Answer from the drawing. Dimensions are ordinates in mm from the lowest x, y and z of the part. Give positions to 0.01 mm unless a question says otherwise; leave off trailing zeros. Loops run counter-clockwise (first coordinate to the right, second up) from the corner with the lowest first, then second, coordinate; pieces in that order, holes last.
(1) Each of these flat-tipped pins is pushed along its axis until it touches: P1, Ø0.7, axis at x = 0.5, y = 22, coming from the +Z side (1 decimal); P2, Ø0.7, axis at x = 0.5, y = 6, coming from the +Z side (1 decimal); P3, Ø0.7, axis at x = 1, z = 22.5, coming from the -Y side. Where does it stop, or does it pass through?
(2) Find section D-D, the plane z = 25.5. Write down the section's boundary in (x, y).
(3) Find section B-B, the plane x = 0.85. State how many separate pieces and enclosed holes the cut face has, then the cut area to 3 significant figures.
(4) Find section A-A, the plane z = 15. Write down the section's boundary in (x, y), then the cut area to 3 significant figures.
(5) Straight lines are drawn through the part: probe 1 along Y at (x, z) = (0.9, 15); probe 2 along Z at (x, y) = (0.15, 6) (1 decimal); probe 3 along Y at (x, z) = (0.3, 20.5) (1 decimal). For each, find the intervals that lie inside material, in ascending order.
(6) Determine the mould class of the marked faces 1 and 2 for opening direction X: pulls with the +X half, pulls with the -X half, needs draft (parallel to the pull), parting line crosses it, or undercut.
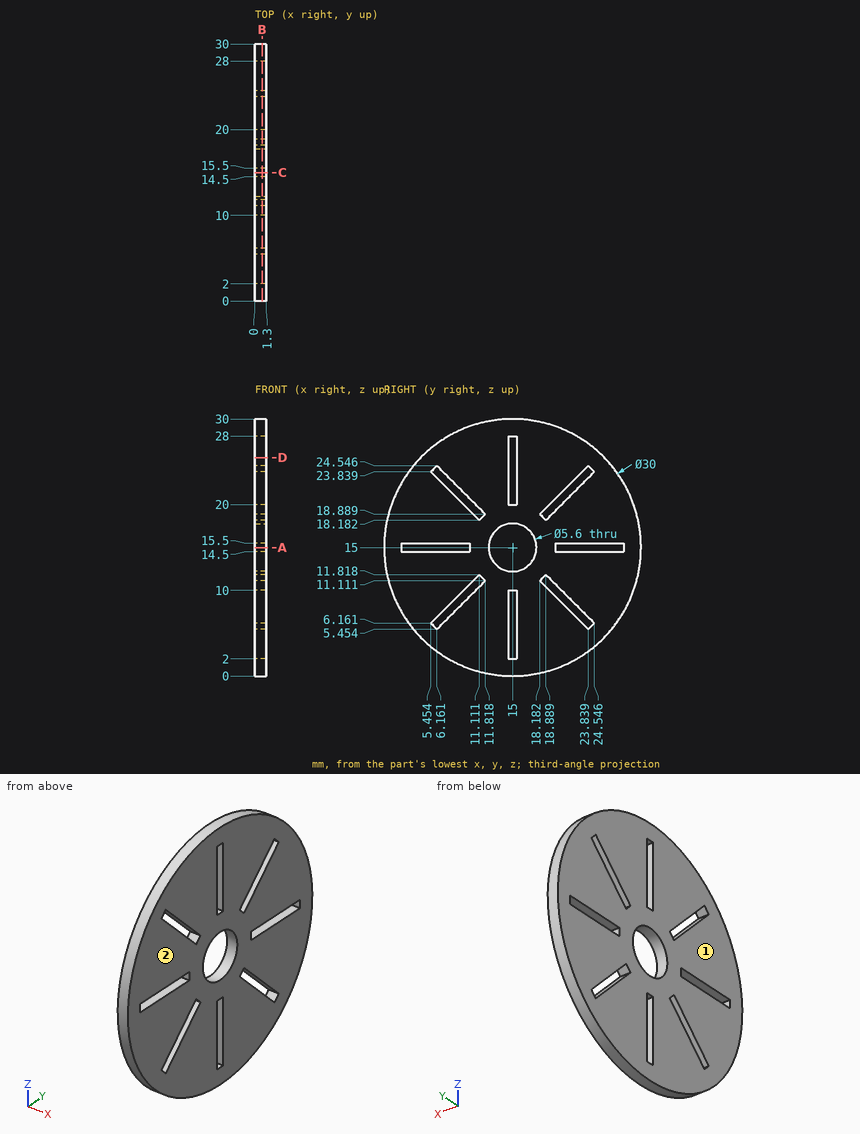
Entries:
1. P1: stops at z = 28.4
1. P2: stops at z = 27.3
1. P3: stops at y = 1.81
2. outline: (0, 4.29) - (1.3, 4.29) - (1.3, 14.5) - (0, 14.5) - close; (0, 15.5) - (1.3, 15.5) - (1.3, 25.71) - (0, 25.71) - close
3. separate pieces: 1
3. enclosed holes: 9
3. area: 618 mm2
4. outline: (0, 0) - (1.3, 0) - (1.3, 2) - (0, 2) - close; (0, 10) - (1.3, 10) - (1.3, 12.2) - (0, 12.2) - close; (0, 17.8) - (1.3, 17.8) - (1.3, 20) - (0, 20) - close; (0, 28) - (1.3, 28) - (1.3, 30) - (0, 30) - close
4. area: 10.9 mm2
5. probe 1: y = 0 to 2, 10 to 12.2, 17.8 to 20, 28 to 30
5. probe 2: z = 3 to 5.6, 6.7 to 14.5, 15.5 to 23.3, 24.4 to 27
5. probe 3: y = 1 to 8.8, 10.2 to 14.5, 15.5 to 19.8, 21.2 to 29
6. face 1: pulls with the -X half
6. face 2: pulls with the +X half
